Input: part model. Units: mm. Frame: model coordinates. A direction names the side the tool comes from. Coordinates: 2 decimals unless noted, no trailing zeros. Order: outer loops, then holes, each group sorted by start corner. A loop starts at its lowest first (then second) coordinate and runs counter-clockwise, first axis right, second up. Notation, with made-up numbers: M -2.5,45.5 L 22.5,45.5 A21 ccw 22.5,66.5 Z; hole C -33,6.25 d5. An arc over 180 degrees is marked long. Answer in a Markdown table with one row per item.
Autodesk Inventor part; units mm, degrees
ref_plane "YZ Plane" through (0, 0, 0) normal (1, 0, 0) x (0, 1, 0)
ref_plane "XZ Plane" through (0, 0, 0) normal (0, 1, 0) x (-1, 0, 0)
ref_plane "XY Plane" through (0, 0, 0) normal (0, 0, 1) x (1, 0, 0)
sketch "Sketch1" plane through (0, 0, 0) normal (0, 1, 0) x (-1, 0, 0)
  circle A0 centre (0, 0) radius 3.5
  circle A1 centre (0, 0) radius 2
  circle A2 centre (0, 0) radius 4.1
  circle A3 centre (0, 0) radius 2.4
  circle A4 centre (0, 0) radius 3.1
  dimension "d0" = 7
  dimension "d1" = 4
  dimension "d2" = 8.2
  dimension "d3" = 0.4
  dimension "d4" = 0.4
extrude "Extrusion1" add sketch "Sketch1" along normal blind 2.5 contours A0 | A3 | A4
extrude "Extrusion2" add sketch "Sketch1" along normal blind 0.6 contours A2
extrude "Extrusion3" cut sketch "Sketch1" along normal blind 0.1 contours A4
extrude "Extrusion4" cut sketch "Sketch1" against normal blind 0.1 from surface at 2.5 contours A4
properties part number "Miniatur Flanschkugellager MF 74 ZZ"
1) Contact query for flat-ended pins moving along their axis: pin 1 (3 mm diameter, centred on x = 0, z = 0, fed in from +Y); pin 2 (1 mm diameter, centred on y = 1.5, z = -0.5, fed in from -X). Output: stop coordinate, or through.
Resolved:
| item | result |
|---|---|
| pin 1 | passes through |
| pin 2 | stops at x = -3.5 |
2) Cut plane D-D, the plane z = -2.5. Output: boundary loops of the cut face in (x, y), and give its area (3 significant figures).
Resolved:
| item | result |
|---|---|
| outline | M -3.25,0 L -1.83,0 L -1.83,0.1 L 1.83,0.1 L 1.83,0 L 3.25,0 L 3.25,0.6 L 2.45,0.6 L 2.45,2.5 L 1.83,2.5 L 1.83,2.4 L -1.83,2.4 L -1.83,2.5 L -2.45,2.5 L -2.45,0.6 L -3.25,0.6 Z |
| area | 12.5 mm2 |
3) Mould query, pull axis X, two halves, no side actions, for faces 1 (the face through (2, 0, 3)), 2 (the face through (-3.233, 1.537, 1.341)), 3 (the face through (0, 1, 2)). Classes: +X half, -X half, draft (parallel to the pull), parting line (faces both ways), or undercut.
Resolved:
| item | result |
|---|---|
| face 1 | draft |
| face 2 | parting line |
| face 3 | undercut |
4) Reachability of faces 4 (the face through (0.534, 0.296, -4.065)), 5 (the face through (-2, 0.1, -2)), 6 (the face through (-2, 2.4, -2)) from +Z, -Z, +X, -X, +Y, -Y: full face, straight path, thin tool, end or side. Return the list, or none.
Resolved:
| item | result |
|---|---|
| face 4 | +Y, -Y |
| face 5 | -Y |
| face 6 | +Y |
5) Cut plane C-C, the plane y = 0.2. Output: boundary loops of the cut face in (x, z).
Resolved:
| item | result |
|---|---|
| outline | C 0,0 d8.2; hole C 0,0 d4 |
6) Cut plane B-B, the plane x = 0. Output: boundary loops of the cut face in (y, z), and give its area (3 significant figures).
Resolved:
| item | result |
|---|---|
| outline | M 0,-4.1 L 0.6,-4.1 L 0.6,-3.5 L 2.5,-3.5 L 2.5,-3.1 L 2.4,-3.1 L 2.4,-2.4 L 2.5,-2.4 L 2.5,-2 L 0,-2 L 0,-2.4 L 0.1,-2.4 L 0.1,-3.1 L 0,-3.1 Z; M 0,2 L 2.5,2 L 2.5,2.4 L 2.4,2.4 L 2.4,3.1 L 2.5,3.1 L 2.5,3.5 L 0.6,3.5 L 0.6,4.1 L 0,4.1 L 0,3.1 L 0.1,3.1 L 0.1,2.4 L 0,2.4 Z |
| area | 7.94 mm2 |
7) Cut plane A-A, the plane z = 0. Output: boundary loops of the cut face in (x, y).
Resolved:
| item | result |
|---|---|
| outline | M -4.1,0 L -3.1,0 L -3.1,0.1 L -2.4,0.1 L -2.4,0 L -2,0 L -2,2.5 L -2.4,2.5 L -2.4,2.4 L -3.1,2.4 L -3.1,2.5 L -3.5,2.5 L -3.5,0.6 L -4.1,0.6 Z; M 2,0 L 2.4,0 L 2.4,0.1 L 3.1,0.1 L 3.1,0 L 4.1,0 L 4.1,0.6 L 3.5,0.6 L 3.5,2.5 L 3.1,2.5 L 3.1,2.4 L 2.4,2.4 L 2.4,2.5 L 2,2.5 Z |
8) Material intervals for probe 1 along Z at (x, y) = (0, 0.75); probe 2 along Y at (x, z) = (-2.5, 1.5); probe 3 along X at (y, z) = (2.05, 1.5), sorted ascending.
Resolved:
| item | result |
|---|---|
| probe 1 | z = -3.5 to -2, 2 to 3.5 |
| probe 2 | y = 0.1 to 2.4 |
| probe 3 | x = -3.16 to -1.32, 1.32 to 3.16 |
